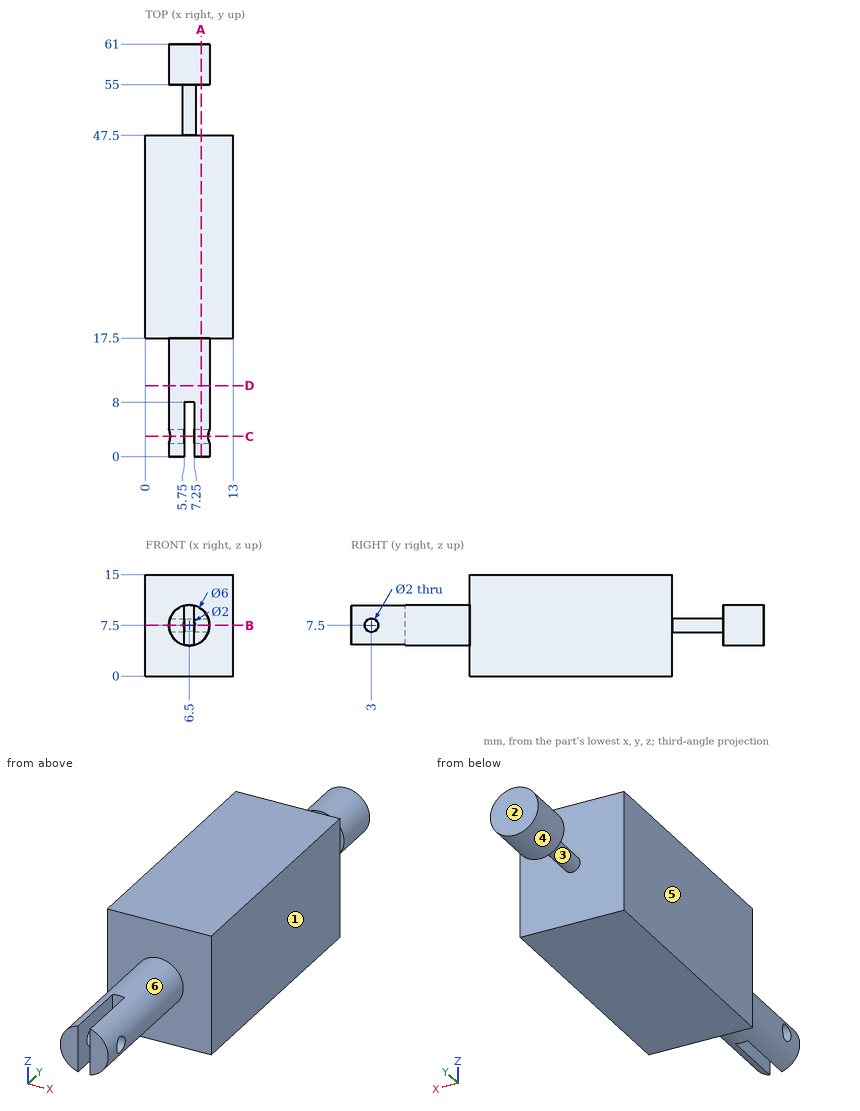
Check sheet for the drawn part. Datum: minimum x, y, z corner. Units: mm. A direction names the side the tool comes from. Give positions to 0.01 mm unless a question says otherwise; leave off trailing zeros. Write each loop counter-clockwise with the first axis right and the second up, starting at its lowest first coordinate (ties: lowest second). Pieces come first, ordered by that corner, then holes. Notation, with made-up numbers: (17.5, 25) - (31.5, 25) arc R28 ccw to (31.5, 44) - close; hole circle Ø9 at (50, -1). An arc over 180 degrees is marked (long way). Put each result on its own line as item: value.
1. Sectioned sample at A-A, the plane x = 8.25. Enter the section's corners in (y, z), plus the area to 3 significant figures.
Ans:
outline: (0, 5.06) - (17.5, 5.06) - (17.5, 0) - (47.5, 0) - (47.5, 15) - (17.5, 15) - (17.5, 9.94) - (0, 9.94) - close; (55, 5.06) - (61, 5.06) - (61, 9.94) - (55, 9.94) - close; hole circle Ø2 at (3, 7.5)
area: 561 mm²
2. Go/stop test with flat-tipped pins: pin 1 (4.5 mm diameter, centred on y = 5.5, z = 6, fed in from +X); pin 2 (1.7 mm diameter, centred on y = 4, z = 7, fed in from -X); pin 3 (1.2 mm diameter, centred on x = 6.5, z = 6.5, fed in from -Y). Record where each tip stops, or that it passes through.
Ans:
pin 1: stops at x = 9.5
pin 2: stops at x = 3.5
pin 3: stops at y = 8
3. Set-up check for the marked faces 4, 5 and 6: record each of +Z, -Z, +X, -X, +Y, -Y from which the full face is reachable in a straight line by a thin tool's end or side.
Ans:
face 4: +Y
face 5: +Z, -Z, -X, +Y, -Y
face 6: -Y
4. Draft check along Y on the marked faces 1, 2 and 3. Enter one of: +Y half, -Y half, draft (parallel to the pull), parting line (faces both ways), or undercut.
Ans:
face 1: draft
face 2: +Y half
face 3: undercut
5. Sectioned sample at B-B, the plane z = 7.5. Enter the section's corners in (x, y), plus the area to 3 significant figures.
Ans:
outline: (0, 17.5) - (3.5, 17.5) - (3.5, 4) - (5.75, 4) - (5.75, 8) - (7.25, 8) - (7.25, 4) - (9.5, 4) - (9.5, 17.5) - (13, 17.5) - (13, 47.5) - (7.5, 47.5) - (7.5, 55) - (9.5, 55) - (9.5, 61) - (3.5, 61) - (3.5, 55) - (5.5, 55) - (5.5, 47.5) - (0, 47.5) - close; (3.5, 0) - (5.75, 0) - (5.75, 2) - (3.5, 2) - close; (7.25, 0) - (9.5, 0) - (9.5, 2) - (7.25, 2) - close
area: 525 mm²
6. Sectioned sample at D-D, the plane y = 10.5. Enter the section's corners in (x, z), plus the area to 3 significant figures.
Ans:
outline: circle Ø6 at (6.5, 7.5)
area: 28.3 mm²
7. Thickness scan on line 1 (Y direction, x = 5, z = 7.5); line 2 (Y direction, x = 0.5, z = 4.25); line 3 (X direction, y = 11.5, z = 9). Record the ranges inside material, lowest first.
Ans:
line 1: y = 0 to 2, 4 to 47.5, 55 to 61
line 2: y = 17.5 to 47.5
line 3: x = 3.9 to 9.1
8. Sectioned sample at C-C, the plane y = 3. Enter the section's corners in (x, z).
Ans:
outline: (3.67, 6.5) arc R3 ccw to (5.75, 4.6) - (5.75, 6.5) - close; (3.67, 8.5) - (5.75, 8.5) - (5.75, 10.4) arc R3 ccw to start; (7.25, 4.6) arc R3 ccw to (9.33, 6.5) - (7.25, 6.5) - close; (7.25, 8.5) - (9.33, 8.5) arc R3 ccw to (7.25, 10.4) - close
